```python
from build123d import *

# Parameters (mm, degrees)
EXTRUDE_1_DEPTH     = 4
SKETCH_2_R          = 3.489709511
EXTRUDE_2_DEPTH     = 1
SKETCH_3_R          = 2.151097983
CUT_EXTRUDE_1_DEPTH = 0.5
FILLET_1_R          = 0.5
FILLET_2_R          = 0.5
SKETCH_4_R          = 3
EXTRUDE_3_DEPTH     = 3
SKETCH_5_R          = 2.5
EXTRUDE_4_DEPTH     = 20


with BuildPart() as part:
    # 草图1 → 凸台-拉伸1 (new body)
    with BuildSketch(Plane.XY):
        with BuildLine():
            ThreePointArc((3.264818601, -2.311051601), (3.989491131, -0.289759403), (3.564498931, 1.815033712))
            add(Edge.make_bspline(
                [(3.564498931, 1.815033712), (0.483839944, 5.460493331), (1.25, 10)],
                knots=[0, 0, 0, 1, 1, 1], degree=2))
            ThreePointArc((1.25, 10), (0, 11.25), (-1.25, 10))
            add(Edge.make_bspline(
                [(-3.564498931, 1.815033712), (-0.483839944, 5.460493331), (-1.25, 10)],
                knots=[0, 0, 0, 1, 1, 1], degree=2))
            ThreePointArc((-3.564498931, 1.815033712), (-3.989491131, -0.289759403), (-3.264818601, -2.311051601))
            add(Edge.make_bspline(
                [(-3.264818601, -2.311051601), (-1.095834513, -4.228126611), (-1.25, -7)],
                knots=[0, 0, 0, 1, 1, 1], degree=2))
            ThreePointArc((-1.25, -7), (0, -8.25), (1.25, -7))
            add(Edge.make_bspline(
                [(3.264818601, -2.311051601), (1.095834513, -4.228126611), (1.25, -7)],
                knots=[0, 0, 0, 1, 1, 1], degree=2))
        make_face()
    extrude(amount=EXTRUDE_1_DEPTH)

    # 草图2 → 凸台-拉伸2 (add)
    with BuildSketch(Plane(origin=(0, 0, 0), x_dir=(-1, 0, 0), z_dir=(0, 0, -1))):
        with Locations((0, 0.098197479)):
            Circle(SKETCH_2_R)
    extrude(amount=EXTRUDE_2_DEPTH)

    # 草图3 → 切除-拉伸1 (cut)
    with BuildSketch(Plane(origin=(0, 0, -1), x_dir=(-1, 0, 0), z_dir=(0, 0, -1))):
        Circle(SKETCH_3_R)
    extrude(amount=-CUT_EXTRUDE_1_DEPTH, mode=Mode.SUBTRACT)

    # 圆角1
    fillet_1_edges = [part.edges().sort_by_distance(p)[0] for p in [
        (2.151097983, 0, -0.5),
    ]]
    fillet(fillet_1_edges, radius=FILLET_1_R - 0.0001)  # a hair under: the kernel refuses the full size

    # 圆角2
    fillet_2_edges = [part.edges().sort_by_distance(p)[0] for p in [
        (3.489709511, 0.098197479, -1),
    ]]
    fillet(fillet_2_edges, radius=FILLET_2_R)

    # 草图4 → 凸台-拉伸3 (add)
    with BuildSketch(Plane.XY.offset(4)):
        Circle(SKETCH_4_R)
    extrude(amount=EXTRUDE_3_DEPTH)

    # 草图5 → 凸台-拉伸4 (add)
    with BuildSketch(Plane.XY.offset(7)):
        Circle(SKETCH_5_R)
    extrude(amount=EXTRUDE_4_DEPTH)


solid = part.part
```
Work out the finished part from the listing and answer in its coordinate system (mm). A direction names the side the tool comes from. Coordinates: 2 decimals unless noted, no trailing zeros. Write each loop counter-clockwise with the first axis right and the second up, starting at its lowest first coordinate (ties: lowest second). Pieces come first, ordered by that corner, then holes.
Q1. Determine the mould class of faces 1 (the face through (-4, 0, 2)), 2 (the face through (0, 0, -0.5)), 3 (the face through (4, 0, 2)), 4 (the face through (0.03, 11.25, 1.97)) for opening direction X: released by +X, released by -X, zero draft, split by the parting line, or undercut.
Q2. A cutting plane is placed at B-B, the plane z = 12.75. Give the vertices of the cut face in (x, y).
Q3. Find the intervals of material crossed by line 1 (Z direction, x = -0.75, y = -4.75); line 2 (Z direction, x = 0.75, y = 2.5); line 3 (Y direction, x = 0, z = 6.75), in increasing order.
Q4. Each of these flat-tipped pins is pushed along its axis until it touches: pin 1 Ø5 at (y, z) = (4, 17.5) entering from -X; pin 2 Ø1.5 at (y, z) = (-1, 2.5) entering from -X; pin 3 Ø1.5 at (x, y) = (3, 9) entering from -Z; pin 4 Ø3 at (y, z) = (-0.5, 6.5) entering from -X. Where does it stop, or does it pass through?
Q5. Which of the six approach directions +Z, -Z, +X, -X, +Y, -Y give full straight-line access (tool end or side, diameter ignored) to faces 5 (the face through (-3.224, -1.238, -0.246)), 6 (the face through (-3, 0, 5)), 7 (the face through (-2, -1.2, -1))?
Findings below:
1. face 1: released by -X
1. face 2: undercut
1. face 3: released by +X
1. face 4: split by the parting line
2. outline: circle Ø5 at (0, 0)
3. line 1: z = 0 to 4
3. line 2: z = -1 to 7
3. line 3: y = -3 to 3
4. pin 1: stops at x = -2
4. pin 2: stops at x = -3.99
4. pin 3: passes through
4. pin 4: stops at x = -3
5. face 5: -Z
5. face 6: +Z
5. face 7: -Z, +X, -X, +Y, -Y
